Autodesk Inventor part; units mm, degrees
ref_plane "YZ Plane" through (0, 0, 0) normal (1, 0, 0) x (0, 1, 0)
ref_plane "XZ Plane" through (0, 0, 0) normal (0, 1, 0) x (-1, 0, 0)
ref_plane "XY Plane" through (0, 0, 0) normal (0, 0, 1) x (1, 0, 0)
sketch "Sketch1" plane through (0, 0, 0) normal (0, 0, 1) x (1, 0, 0)
  circle A0 centre (0, 0) radius 1.75
  circle A1 centre (0, 0) radius 3.5
  circle A2 centre (0, 0) radius 2.5
  dimension "d0" = 3.5
  dimension "d1" = 7
  dimension "d9" = 5
extrude "Extrusion1" add sketch "Sketch1" along normal blind 9 contours A2
extrude "Extrusion2" add sketch "Sketch1" along normal blind 1 contours A1 | A2
sketch "Sketch2" plane through (0, 0, 9) normal (0, 0, 1) x (1, 0, 0)
  circle A0 centre (0, 0) radius 3.5
  circle A1 centre (0, 0) radius 1.75
  dimension "d6" = 7
  dimension "d10" = 3.5
extrude "Extrusion3" add sketch "Sketch2" against normal blind 1
sketch "Sketch3" plane through (0, 0, 0) normal (0, 0, -1) x (-1, 0, 0)
  circle A0 centre (0, 0) radius 2
  circle A1 centre (0, 0) radius 1.75
  dimension "d11" = 4
  dimension "d12" = 3.5
extrude "Extrusion4" add sketch "Sketch3" along normal blind 0.5
sketch "Sketch4" plane through (0, 0, 9) normal (0, 0, 1) x (1, 0, 0)
  circle A0 centre (0, 0) radius 1.75
  circle A1 centre (0, 0) radius 1.75
  circle A2 centre (0, 0) radius 2
  dimension "d15" = 3.5
  dimension "d16" = 4
extrude "Extrusion5" add sketch "Sketch4" along normal blind 0.5
properties part number "GuidingPulley"
Geometry: final body of the model. Coordinates: model frame, mm. A direction names the side the tool comes from. Round coordinates to 2 decimals unless told otherwise and drop trailing zeros. Order: outer loops, then holes, each group sorted by start corner. A loop starts at its lowest first (then second) coordinate and runs counter-clockwise, first axis right, second up. Notation, with made-up numbers: (-18, -37.75) -> (41, -37.75) arc R20 ccw to (41, -9.75) -> close; hole circle Ø10 at (51.25, 75.25). An arc over 180 degrees is marked (long way). Write each question's results on one line, items separated by ' | '.
Q1. Pull-direction query (Z, two-part tool) for faces 1 (the face through (0.434, 1.952, -0.246)), 2 (the face through (2, -2, 0)), 3 (the face through (-0.54, 2.44, 4.45)); classes: released by +Z, released by -Z, zero draft, split by the parting line, or undercut.
Response values:
face 1: zero draft | face 2: released by -Z | face 3: undercut
Q2. Access query for faces 4 (the face through (-0.434, 1.952, 9.246)), 5 (the face through (2, -2, 8)), 6 (the face through (3.233, -1.341, 8.507)). Directions: +Z, -Z, +X, -X, +Y, -Y. A direction counts if a zero-diameter tool reaches every point of the face in a straight line with its end or side. Return the directions, or none.
Response values:
face 4: +Z | face 5: none | face 6: +Z, -Z
Q3. Section query A-A (x = 0). Output: boundary loops of the cut face in (y, z).
Response values:
outline: (-3.5, 0) -> (-2, 0) -> (-2, -0.5) -> (-1.75, -0.5) -> (-1.75, 9.5) -> (-2, 9.5) -> (-2, 9) -> (-3.5, 9) -> (-3.5, 8) -> (-2.5, 8) -> (-2.5, 1) -> (-3.5, 1) -> close; (1.75, -0.5) -> (2, -0.5) -> (2, 0) -> (3.5, 0) -> (3.5, 1) -> (2.5, 1) -> (2.5, 8) -> (3.5, 8) -> (3.5, 9) -> (2, 9) -> (2, 9.5) -> (1.75, 9.5) -> close
Q4. Section query D-D (y = -2.25). Output: boundary loops of the cut face in (x, z), and give its area (3 significant figures).
Response values:
outline: (-2.68, 0) -> (2.68, 0) -> (2.68, 1) -> (1.09, 1) -> (1.09, 8) -> (2.68, 8) -> (2.68, 9) -> (-2.68, 9) -> (-2.68, 8) -> (-1.09, 8) -> (-1.09, 1) -> (-2.68, 1) -> close | area: 26.0 mm²
Q5. Section query C-C (z = 2). Output: boundary loops of the cut face in (x, y).
Response values:
outline: circle Ø5 at (0, 0); hole circle Ø3.5 at (0, 0)
Q6. Pin query (flat end, axial travel): pin 1 Ø2 at (x, z) = (1.5, 3.5) entering from -Y; pin 2 Ø1.5 at (y, z) = (1, 5.5) entering from -X. Return the tip coordinate at first contact, or that it passes through.
Response values:
pin 1: y = -2.45 | pin 2: x = -2.49
Q7. Ray query, line 1 along Z through (x, y) = (-2.5, -0.5); line 2 along Y through (x, z) = (0, 9.35); line 3 along Y through (x, z) = (0, 7.25). Return the intervals inside material, ascending.
Response values:
line 1: 0 to 1, 8 to 9 | line 2: -2 to -1.75, 1.75 to 2 | line 3: -2.5 to -1.75, 1.75 to 2.5
